Geometry check sheet. Reference: the model listing, model coordinates, mm. Coordinates: 2 decimals unless noted, no trailing zeros. Write each loop counter-clockwise with the first axis right and the second up, starting at its lowest first coordinate (ties: lowest second). Pieces come first, ordered by that corner, then holes. Notation, with made-up numbers: (-35.75, 87.5) -> (-23.75, 87.5) arc R12 cw to (-23.75, 103.5) -> close; hole circle Ø9 at (25.5, -23). An arc over 180 degrees is marked (long way). Answer in a Markdown table with one row per item. Add a question column.
1. Cross-section at A-A on y = -113. Record the cut outline in (x, z), and give its area (3 significant figures).
2. Cross-section at C-C on x = -141. Record the cut outline in (y, z).
3. Cross-section at B-B on z = 3.75. Record the cut outline in (x, y), and give its area (3 significant figures).
4. Depth check by flat-ended pin: P1, Ø9.5, axis at y = 165.5, z = 14, coming from the -X side; P2, Ø10, axis at x = 92, y = 61, coming from the -Z side. Enter the tip coordinate at first touch or a pass-through.
5. Scan lines: L1, parallel to Y at x = -111, z = 1.25; L2, parallel to Y at x = -46.5, z = 15; L3, parallel to X at y = -143, z = 9. Record each from-to range of solid material in increasing order. Write a range as from..to.
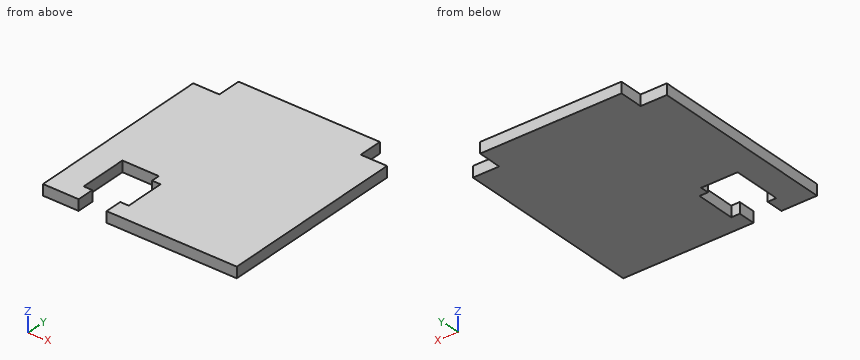
```python
from build123d import *

# Parameters (mm, degrees)
ESQUISSE1_W             = 340
ESQUISSE1_H             = 372.5
BOSS_EXTRU_1_DEPTH      = 19
ESQUISSE2_W             = 46
ESQUISSE2_H             = 42
ENL_V_MAT_EXTRU_1_DEPTH = 253.883495903
ESQUISSE4_W             = 79
ESQUISSE4_H             = 100
ENL_V_MAT_EXTRU_2_DEPTH = 30
ESQUISSE5_W             = 15
ESQUISSE5_H             = 15
BOSS_EXTRU_2_DEPTH      = 19
ESQUISSE6_W             = 49
ESQUISSE6_H             = 15
ENL_V_MAT_EXTRU_3_DEPTH = 20


with BuildPart() as part:
    # Esquisse1 → Boss.-Extru.1 (new body)
    with BuildSketch(Plane.XY):
        Rectangle(ESQUISSE1_W, ESQUISSE1_H)
    extrude(amount=BOSS_EXTRU_1_DEPTH)

    # Esquisse2 → Enlèv. mat.-Extru.1 (cut, through all)
    with BuildSketch(Plane.XY.offset(19)):
        with Locations((-147, 165.25)):
            Rectangle(ESQUISSE2_W, ESQUISSE2_H)
        with Locations((147, 165.25)):
            Rectangle(ESQUISSE2_W, ESQUISSE2_H)
    extrude(amount=-ENL_V_MAT_EXTRU_1_DEPTH, mode=Mode.SUBTRACT)

    # Esquisse4 → Enlèv. mat.-Extru.2 (cut)
    with BuildSketch(Plane.XY.offset(19)):
        with Locations((-83, -121.25)):
            Rectangle(ESQUISSE4_W, ESQUISSE4_H)
    extrude(amount=-ENL_V_MAT_EXTRU_2_DEPTH, mode=Mode.SUBTRACT)

    # Esquisse5 → Boss.-Extru.2 (add)
    with BuildSketch(Plane.XY.offset(19)):
        with Locations((-51, -163.75)):
            Rectangle(ESQUISSE5_W, ESQUISSE5_H)
        with Locations((-115, -163.75)):
            Rectangle(ESQUISSE5_W, ESQUISSE5_H)
        with Locations((-51, -78.75)):
            Rectangle(ESQUISSE5_W, ESQUISSE5_H)
    extrude(amount=-BOSS_EXTRU_2_DEPTH)

    # Esquisse6 → Enlèv. mat.-Extru.3 (cut)
    with BuildSketch(Plane.XY.offset(19)):
        with Locations((-83, -178.75)):
            Rectangle(ESQUISSE6_W, ESQUISSE6_H)
    extrude(amount=-ENL_V_MAT_EXTRU_3_DEPTH, mode=Mode.SUBTRACT)


solid = part.part
```
Results found:
| question | item | result |
|---|---|---|
| 1 | outline | (-170, 0) -> (-122.5, 0) -> (-122.5, 19) -> (-170, 19) -> close; (-43.5, 0) -> (170, 0) -> (170, 19) -> (-43.5, 19) -> close |
| 1 | area | 4,960 mm^2 |
| 2 | outline | (-186.25, 0) -> (144.25, 0) -> (144.25, 19) -> (-186.25, 19) -> close |
| 3 | outline | (-170, -186.25) -> (-107.5, -186.25) -> (-107.5, -156.25) -> (-122.5, -156.25) -> (-122.5, -71.25) -> (-58.5, -71.25) -> (-58.5, -86.25) -> (-43.5, -86.25) -> (-43.5, -156.25) -> (-58.5, -156.25) -> (-58.5, -186.25) -> (170, -186.25) -> (170, 144.25) -> (124, 144.25) -> (124, 186.25) -> (-124, 186.25) -> (-124, 144.25) -> (-170, 144.25) -> close |
| 3 | area | 115,000 mm^2 |
| 4 | P1 | stops at x = -124 |
| 4 | P2 | stops at z = 0 |
| 5 | L1 | y = -186.25..-156.25, -71.25..186.25 |
| 5 | L2 | y = -186.25..-156.25, -86.25..186.25 |
| 5 | L3 | x = -170..-122.5, -43.5..170 |
